from build123d import *

# Parameters (mm, degrees)
MODEL_R         = 1.5
MODEL_R_2       = 1.15
MODEL_R_3       = 1
MODEL_W         = 8.161843832
MODEL_H         = 10.8383371
EXTRUDE_1_DEPTH = 3


with BuildPart() as part:
    # Model → 凸台-拉伸1 (new body)
    with BuildSketch(Plane.XY):
        with BuildLine():
            Line((-43.059438732, 38.219900225), (-48.592321023, 32.687017934))
            Line((-48.592321023, 32.687017934), (-48.592321023, 12.182501991))
            Line((-48.592321023, 12.182501991), (-36.344324073, 0))
            Line((-36.344324073, 0), (36.344324073, 0))
            Line((36.344324073, 0), (48.592321023, 12.182501991))
            Line((48.592321023, 12.182501991), (48.592321023, 32.687017934))
            Line((48.592321023, 32.687017934), (43.059438732, 38.219900225))
            Line((43.059438732, 38.219900225), (43.059438732, 68.896640242))
            Line((43.059438732, 68.896640242), (27.8, 84.156078975))
            Line((27.8, 84.156078975), (27.8, 110))
            ThreePointArc((27.8, 110), (24.5, 113.3), (21.2, 110))
            Line((21.2, 110), (21.2, 83.314119419))
            Line((21.2, 83.314119419), (16.324508054, 78.438627474))
            Line((16.324508054, 78.438627474), (0, 90.063749844))
            Line((0, 90.063749844), (-16.324508054, 78.438627474))
            Line((-16.324508054, 78.438627474), (-21.2, 83.314119419))
            Line((-21.2, 83.314119419), (-21.2, 110))
            ThreePointArc((-21.2, 110), (-24.5, 113.3), (-27.8, 110))
            Line((-27.8, 110), (-27.8, 84.156078975))
            Line((-27.8, 84.156078975), (-43.059438732, 68.896640242))
            Line((-43.059438732, 68.896640242), (-43.059438732, 38.219900225))
        make_face()
        with Locations((-24.5, 110)):
            Circle(MODEL_R, mode=Mode.SUBTRACT)
        with Locations(Location((8, 79.632653547, 0), (0, 0, 180))):
            Circle(MODEL_R_2, mode=Mode.SUBTRACT)
        with Locations(Location((36.990563228, 5.05084864, 0), (0, 0, 180))):
            Circle(MODEL_R, mode=Mode.SUBTRACT)
        with Locations(Location((37.227006719, 69.050411877, 0), (0, 0, 180))):
            Circle(MODEL_R, mode=Mode.SUBTRACT)
        with Locations((-41.292321023, 13.694034445)):
            Circle(MODEL_R_3, mode=Mode.SUBTRACT)
        with Locations((-41.292321023, 31.294034445)):
            Circle(MODEL_R_3, mode=Mode.SUBTRACT)
        with Locations(Location((41.292321023, 31.294034445, 0), (0, 0, 180))):
            Circle(MODEL_R_3, mode=Mode.SUBTRACT)
        with Locations((-37.227006719, 69.050411877)):
            Circle(MODEL_R, mode=Mode.SUBTRACT)
        with Locations((-36.990563228, 5.05084864)):
            Circle(MODEL_R, mode=Mode.SUBTRACT)
        with Locations(Location((41.292321023, 13.694034445, 0), (0, 0, 180))):
            Circle(MODEL_R_3, mode=Mode.SUBTRACT)
        with Locations((-8, 79.632653547)):
            Circle(MODEL_R_2, mode=Mode.SUBTRACT)
        with Locations(Location((24.5, 110, 0), (0, 0, 180))):
            Circle(MODEL_R, mode=Mode.SUBTRACT)
        with Locations((39.518535679, 21.492278657)):
            Rectangle(MODEL_W, MODEL_H, mode=Mode.SUBTRACT)
        with Locations((-39.518535679, 21.492278657)):
            Rectangle(MODEL_W, MODEL_H, mode=Mode.SUBTRACT)
        with BuildLine():
            Line((-32.294540613, 70.550411877), (-5.361487625, 70.550411877))
            ThreePointArc((-5.361487625, 70.550411877), (-3.861487625, 69.050411877), (-5.361487625, 67.550411877))
            Line((-5.361487625, 67.550411877), (-32.294540613, 67.550411877))
            ThreePointArc((-32.294540613, 67.550411877), (-33.794540613, 69.050411877), (-32.294540613, 70.550411877))
        make_face(mode=Mode.SUBTRACT)
        with BuildLine():
            Line((-35.727006719, 62.728595156), (-35.727006719, 37.828225412))
            ThreePointArc((-35.727006719, 37.828225412), (-37.227006719, 36.328225412), (-38.727006719, 37.828225412))
            Line((-38.727006719, 37.828225412), (-38.727006719, 62.728595156))
            ThreePointArc((-38.727006719, 62.728595156), (-37.227006719, 64.228595156), (-35.727006719, 62.728595156))
        make_face(mode=Mode.SUBTRACT)
        with BuildLine():
            Line((-30.622515674, 63.263136287), (-7.472898393, 40.435705899))
            ThreePointArc((-7.472898393, 40.435705899), (-7.45803348, 38.314437638), (-9.579301741, 38.299572725))
            Line((-9.579301741, 38.299572725), (-32.728919021, 61.127003113))
            ThreePointArc((-32.728919021, 61.127003113), (-32.743783934, 63.248271374), (-30.622515674, 63.263136287))
        make_face(mode=Mode.SUBTRACT)
        with BuildLine():
            Line((-7.627164767, 30.804285944), (-30.776782047, 10.299770001))
            ThreePointArc((-30.776782047, 10.299770001), (-32.894218954, 10.428070228), (-32.765918727, 12.545507134))
            Line((-32.765918727, 12.545507134), (-9.616301447, 33.050023077))
            ThreePointArc((-9.616301447, 33.050023077), (-7.49886454, 32.92172285), (-7.627164767, 30.804285944))
        make_face(mode=Mode.SUBTRACT)
        with BuildLine():
            Line((-32.765918727, 6.55084864), (-2.834717307, 6.55084864))
            ThreePointArc((-2.834717307, 6.55084864), (-1.334717307, 5.05084864), (-2.834717307, 3.55084864))
            Line((-2.834717307, 3.55084864), (-32.765918727, 3.55084864))
            ThreePointArc((-32.765918727, 3.55084864), (-34.265918727, 5.05084864), (-32.765918727, 6.55084864))
        make_face(mode=Mode.SUBTRACT)
        with BuildLine():
            Line((32.765918727, 6.55084864), (2.834717307, 6.55084864))
            ThreePointArc((2.834717307, 6.55084864), (1.334717307, 5.05084864), (2.834717307, 3.55084864))
            Line((2.834717307, 3.55084864), (32.765918727, 3.55084864))
            ThreePointArc((32.765918727, 3.55084864), (34.265918727, 5.05084864), (32.765918727, 6.55084864))
        make_face(mode=Mode.SUBTRACT)
        with BuildLine():
            Line((7.627164767, 30.804285944), (30.776782047, 10.299770001))
            ThreePointArc((30.776782047, 10.299770001), (32.894218954, 10.428070228), (32.765918727, 12.545507134))
            Line((32.765918727, 12.545507134), (9.616301447, 33.050023077))
            ThreePointArc((9.616301447, 33.050023077), (7.49886454, 32.92172285), (7.627164767, 30.804285944))
        make_face(mode=Mode.SUBTRACT)
        with BuildLine():
            Line((35.727006719, 62.728595156), (35.727006719, 37.828225412))
            ThreePointArc((35.727006719, 37.828225412), (37.227006719, 36.328225412), (38.727006719, 37.828225412))
            Line((38.727006719, 37.828225412), (38.727006719, 62.728595156))
            ThreePointArc((38.727006719, 62.728595156), (37.227006719, 64.228595156), (35.727006719, 62.728595156))
        make_face(mode=Mode.SUBTRACT)
        with BuildLine():
            Line((30.622515674, 63.263136287), (7.472898393, 40.435705899))
            ThreePointArc((7.472898393, 40.435705899), (7.45803348, 38.314437638), (9.579301741, 38.299572725))
            Line((9.579301741, 38.299572725), (32.728919021, 61.127003113))
            ThreePointArc((32.728919021, 61.127003113), (32.743783934, 63.248271374), (30.622515674, 63.263136287))
        make_face(mode=Mode.SUBTRACT)
        with BuildLine():
            Line((32.294540613, 70.550411877), (5.361487625, 70.550411877))
            ThreePointArc((5.361487625, 70.550411877), (3.861487625, 69.050411877), (5.361487625, 67.550411877))
            Line((5.361487625, 67.550411877), (32.294540613, 67.550411877))
            ThreePointArc((32.294540613, 67.550411877), (33.794540613, 69.050411877), (32.294540613, 70.550411877))
        make_face(mode=Mode.SUBTRACT)
        with BuildLine():
            Line((1.5, 62.1950697), (1.5, 13.888925857))
            ThreePointArc((1.5, 13.888925857), (0, 12.388925857), (-1.5, 13.888925857))
            Line((-1.5, 13.888925857), (-1.5, 62.1950697))
            ThreePointArc((-1.5, 62.1950697), (0, 63.6950697), (1.5, 62.1950697))
        make_face(mode=Mode.SUBTRACT)
    extrude(amount=EXTRUDE_1_DEPTH)


solid = part.part
Work out the finished part from the listing and answer in its coordinate system (mm). A direction names the side the tool comes from. Give positions to 0.01 mm unless a question says otherwise; leave off trailing zeros. Order: outer loops, then holes, each group sorted by start corner. A loop starts at its lowest first (then second) coordinate and runs counter-clockwise, first axis right, second up. Notation, with made-up numbers: (79, 15) - (83, 15) arc R28 cw to (83, 42) - close; hole circle Ø11 at (48, 47). An arc over 180 degrees is marked (long way). Answer as CSV lines item,"result". Start each with the question number.
Q1. For faces 1 (the face through (-43.059, 54, 1)), 2 (the face through (-19, 70.55, 1)), 3 (the face through (-18.728, 80.842, 1.479)), determine the directions among +Z, -Z, +X, -X, +Y, -Y from which every point of the face is accessible in a straight line to the end or side of a thin tool.
Q2. The part is cut by section A-A (x = 24.5). Write down the section's boundary in (y, z), then the cut area to 3 significant figures.
Q3. The mould has two halves that part along Y. Classify faces 4 (the face through (21.2, 97, 1)), 5 (the face through (8.249, 80.755, 1.479)), 6 (the face through (-35.323, 76.633, 1.479)): +Y half, -Y half, draft (parallel to the pull), parting line (faces both ways), or undercut.
Q4. The part is cut by section C-C (z = 1.55). Give the number of separate pieces and of enclosed holes in the cut face, then the cut area to 3 significant figures.
Q5. Given pin 1 Ø1.8 at (x, y) = (-41.29, 13.69) entering from -Z; pin 2 Ø1 at (x, z) = (-34, 1.5) entering from +Y; pin 3 Ø1.5 at (x, z) = (-19, 1.5) entering from +Y, each flat-ended and moving along its own axis, determine where each tip first touches the part or whether it passes through.
Q6. The part is cut by section B-B (y = 57). Write down the section's boundary in (x, z).
Q7. Find the intervals of material crossed by L1, parallel to X at y = 110, z = 1.5; L2, parallel to X at y = 30, z = 0.6; L3, parallel to X at y = 98, z = 1.35, in increasing order. Write a range as [from, to].
Check result:
1,face 1,"+Z, -Z, -X, +Y"
1,face 2,"+Z, -Z"
1,face 3,"+Z, -Z, +Y"
2,outline,"(0, 0) - (3.55, 0) - (3.55, 3) - (0, 3) - close; (6.55, 0) - (15.86, 0) - (15.86, 3) - (6.55, 3) - close; (19.87, 0) - (53.01, 0) - (53.01, 3) - (19.87, 3) - close; (57.23, 0) - (67.55, 0) - (67.55, 3) - (57.23, 3) - close; (70.55, 0) - (108.5, 0) - (108.5, 3) - (70.55, 3) - close; (111.5, 0) - (113.3, 0) - (113.3, 3) - (111.5, 3) - close"
2,area,"288 mm²"
3,face 4,"draft"
3,face 5,"undercut"
3,face 6,"+Y half"
4,separate pieces,"1"
4,enclosed holes,"25"
4,area,"6,270 mm²"
5,pin 1,"passes through"
5,pin 2,"stops at y = 78.46"
5,pin 3,"stops at y = 81.86"
6,outline,"(-43.06, 0) - (-38.73, 0) - (-38.73, 3) - (-43.06, 3) - close; (-35.73, 0) - (-28.54, 0) - (-28.54, 3) - (-35.73, 3) - close; (-24.27, 0) - (-1.5, 0) - (-1.5, 3) - (-24.27, 3) - close; (1.5, 0) - (24.27, 0) - (24.27, 3) - (1.5, 3) - close; (28.54, 0) - (35.73, 0) - (35.73, 3) - (28.54, 3) - close; (38.73, 0) - (43.06, 0) - (43.06, 3) - (38.73, 3) - close"
7,L1,"x = [-27.8, -26], [-23, -21.2], [21.2, 23], [26, 27.8]"
7,L2,"x = [-48.59, -13.06], [-8.54, -1.5], [1.5, 8.54], [13.06, 48.59]"
7,L3,"x = [-27.8, -21.2], [21.2, 27.8]"
